Here's the drawing with two shaded views (mm, measured from the low corner). I have some questions. A direction names the side the tool comes from. Coordinates: 2 decimals unless noted, no trailing zeros. Write each loop counter-clockwise with the first axis right and the second up, starting at its lowest first coordinate (ties: lowest second). Pieces come first, ordered by that corner, then holes. Notation, with made-up numbers: M 28.25,38.25 L 32.25,38.25 A15 cw 32.25,54.25 Z; hole C 67.5,70.5 d11. An arc over 180 degrees is marked long. Answer as CSV lines item,"result". Start each with the question number.
Item 1: If I drill on line 1 along Y through (x, z) = (6, 2.75); line 2 along X through (y, z) = (3.75, 0.7); line 3 along Y through (x, z) = (36, 0.75), over which ranges is the centre line in solid material (lowest first)? Write a range as [from, to].
Item 2: Suppose I cut it at D-D, the plane x = 7.5. Write out the boundary of the cut face in (y, z).
Item 3: On a 3-axis mill with a long thin cutter (end or side, diameter ignored), from which of +Z, -Z, +X, -X, +Y, -Y can I reach the whole of each face in a straight line? I mean the marked faces 1 and 2. Say none if no direction works.
Item 4: I'm going to push flat-ended pins straight in: P1, Ø3, axis at x = 7, y = 5, coming from the +Z side; P2, Ø3, axis at x = 6.5, y = 5.5, coming from the -Z side; P3, Ø2.5, axis at x = 20, y = 5, coming from the -Z side. Where does each tip first touch, or does it pass through?
Item 5: Suppose I cut it at C-C, the plane x = 34. Write out the boundary of the cut face in (y, z).
Item 6: Suppose I cut it at B-B, the plane x = 20. Write out the boundary of the cut face in (y, z), and give its area (3 significant figures).
Item 7: Suppose I cut it at A-A, the plane z = 1.75. State how many separate pieces and enclosed holes the cut face has, and give its area (3 significant figures).
Item 8: We'd pull the mould along X, two halves only. Please class the marked faces 3, 4 and 5: +X half, -X half, draft (parallel to the pull), parting line (faces both ways), or undercut.
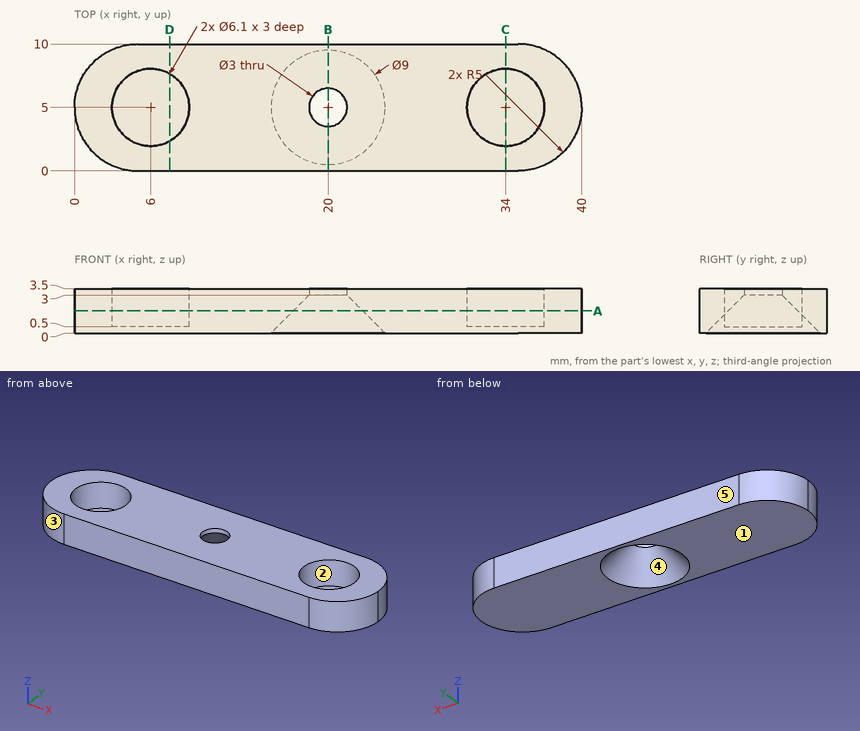
Ans:
1,line 1,"y = [0, 1.95], [8.05, 10]"
1,line 2,"x = [0.16, 3.22], [8.78, 16.41], [23.59, 31.22], [36.78, 39.84]"
1,line 3,"y = [0.1, 2.7], [7.3, 9.9]"
2,outline,"M 0,0 L 10,0 L 10,3.5 L 7.66,3.5 L 7.66,0.5 L 2.34,0.5 L 2.34,3.5 L 0,3.5 Z"
3,face 1,"-Z, +X, -X, +Y, -Y"
3,face 2,"+Z"
4,P1,"stops at z = 0.5"
4,P2,"stops at z = 0"
4,P3,"passes through"
5,outline,"M 0,0 L 10,0 L 10,3.5 L 8.05,3.5 L 8.05,0.5 L 1.95,0.5 L 1.95,3.5 L 0,3.5 Z"
6,outline,"M 0,0 L 0.5,0 L 3.5,3 L 3.5,3.5 L 0,3.5 Z; M 6.5,3 L 9.5,0 L 10,0 L 10,3.5 L 6.5,3.5 Z"
6,area,"15.5 mm^2"
7,separate pieces,"1"
7,enclosed holes,"3"
7,area,"296 mm^2"
8,face 3,"-X half"
8,face 4,"undercut"
8,face 5,"draft"
